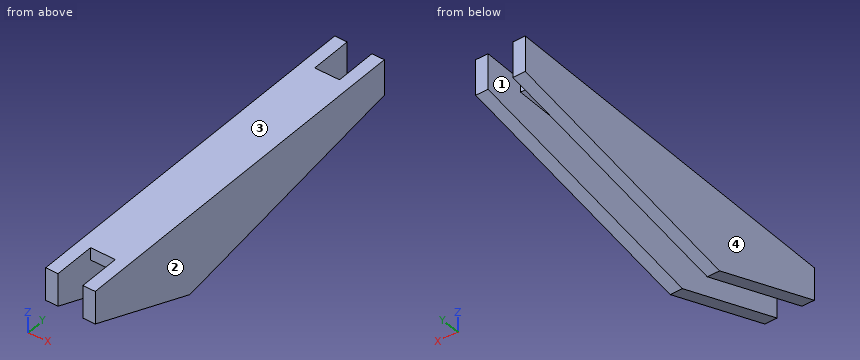
Autodesk Inventor part; units mm, degrees
ref_plane "YZ Plane" through (0, 0, 0) normal (1, 0, 0) x (0, 1, 0)
ref_plane "XZ Plane" through (0, 0, 0) normal (0, 1, 0) x (-1, 0, 0)
ref_plane "XY Plane" through (0, 0, 0) normal (0, 0, 1) x (1, 0, 0)
sketch "BoundingBox" plane through (0, 0, 0) normal (1, 0, 0) x (0, 1, 0)
  line L0 (434.8115, 24.0504) -> (-18, 24.0504)
  line L1 (-18, 24.0504) -> (-18, -15.6719)
  line L2 (-18, -15.6719) -> (130.2861, -72.3729)
  line L3 (130.2861, -72.3729) -> (434.8115, -19.2646)
  line L4 (434.8115, -19.2646) -> (434.8115, 24.0504)
  point P0 (0, 0)
  point P1 (417.3115, 0.6447)
  point P2 (-18, 4.1892)
  dimension "d5" = 24.0504
  dimension "d6" = 4.1893
  dimension "d7" = 110.926
  dimension "d8" = 452.8115
  dimension "d9" = 39.7223
  dimension "d10" = 43.315
  dimension "d11" = 99.893
  dimension "d12" = 56.7009
  dimension "d13" = 17.5
  dimension "d14" = 23.4057
extrude "BoundingBoxFeature" add sketch "BoundingBox" along normal mid plane 60
sketch "ForearmSpace" plane through (0, 0, 0) normal (0, 0, 1) x (1, 0, 0)
  line L0 (15, 142.9861) -> (-15, 142.9861)
  line L1 (-15, 142.9861) -> (-15, 434.8115)
  line L2 (-15, 434.8115) -> (15, 434.8115)
  line L3 (15, 434.8115) -> (15, 142.9861)
  line L4 (-30, 434.8115) -> (30, 434.8115)
  line L5 (0, -86.9623) -> (0, 521.7738)
  line L6 (30, 130.2861) -> (30, 434.8115)
  line L7 (-30, 130.2861) -> (30, 130.2861)
  line L8 (-30, 434.8115) -> (-30, 130.2861)
  line L9 (15, 142.9861) -> (-15, 142.9861)
  line L10 (-15, 142.9861) -> (-15, -18)
  line L11 (-15, -18) -> (15, -18)
  line L12 (15, -18) -> (15, 142.9861)
  line L13 (-30, -18) -> (30, -18)
  point P0 (0, 0)
  point P1 (-30, 282.5488)
  point P2 (0, 142.9861)
  dimension "d19" = 12.7
  dimension "d21" = 30
extrude "ForearmCutFeature" cut sketch "ForearmSpace" along normal through all both and the other way through all contours L12 L7 L5 L0 | L0 L5 L2 L3 | L5 L7 L10 L0 | L0 L1 L2 L5 | L12 L11 L5 L7 | L5 L11 L10 L7
sketch "Sketch4" plane through (30, 0, 0) normal (1, 0, 0) x (0, 0, -1)
  line L0 (-24.0504, 434.8115) -> (-24.0504, -18)
  line L1 (-24.0504, 32.8) -> (-9.0504, 32.8)
  line L2 (-9.0504, 32.8) -> (-9.0504, 384.0115)
  line L3 (-9.0504, 384.0115) -> (-24.0504, 384.0115)
  line L4 (-24.0504, 384.0115) -> (-24.0504, 32.8)
  line L5 (-24.0504, -18) -> (15.6719, -18)
  line L6 (19.2646, 434.8115) -> (-24.0504, 434.8115)
  point P0 (0, 0)
  dimension "d25" = 15
  dimension "d26" = 50.8
  dimension "d27" = 50.8
extrude "Extrusion3" add sketch "Sketch4" against normal up to surface (45 mm away)
properties part number "UpperArmBoundingBox"
Build history of the part. All positions in model axes, mm. Face numbers are marked on the shaded views. Give positions to 0.01 mm unless a question says otherwise; leave off trailing zeros. Loops run counter-clockwise (first coordinate to the right, second up) from the corner with the lowest first, then second, coordinate; pieces in that order, holes last. Notation, with made-up numbers: (-7, 55) -> (3, 55) arc R26 cw to (3, 88) -> close; hole circle Ø6 at (-9.75, -2). An arc over 180 degrees is marked (long way). One line per question, with ' | ' between items. Start each with the question number.
1) Probe L1, parallel to X at y = 266.5, z = -20.5; L2, parallel to Z at x = 11.5, y = 371.5; L3, parallel to Z at x = 18, y = 395.5. List the from-to ranges inside material, lowest first.
2) Two-plate mould, pull along X, no slides. Class the marked faces 1, 2, 3 and 4: released by +X, released by -X, zero draft, split by the parting line, or undercut.
3) Pin check, flat tips, straight feed: pin 1 (4 mm diameter, centred on x = -3.5, y = 264, fed in from -Z); pin 2 (12 mm diameter, centred on x = -2.5, z = 15.5, fed in from -Y); pin 3 (8 mm diameter, centred on y = 322, z = -39, fed in from -X); pin 4 (16.5 mm diameter, centred on x = 5, z = 13.5, fed in from +Y). Stop position of each tip, or through.
4) Cut at D-D (y = 177.5). Give the cut face in (x, z), plus the area to 3 significant figures.
5) Cut at A-A (z = -8). Give the cut face in (x, y), plus the area to 3 significant figures.
6) Cut at C-C (x = 20.5). Give the cut face in (y, z).
7) Cut at B-B (z = 16). Give the cut face in (x, y).
Return value:
1) L1: -30 to -15, 15 to 30 | L2: 9.05 to 24.05 | L3: -26.12 to 24.05
2) face 1: undercut | face 2: released by +X | face 3: zero draft | face 4: released by -X
3) pin 1: z = 9.05 | pin 2: y = 32.8 | pin 3: x = -30 | pin 4: y = 384.01
4) outline: (-30, -64.14) -> (-15, -64.14) -> (-15, 9.05) -> (15, 9.05) -> (15, -64.14) -> (30, -64.14) -> (30, 24.05) -> (-30, 24.05) -> close | area: 3,100 mm^2
5) outline: (-30, -18) -> (-15, -18) -> (-15, 434.81) -> (-30, 434.81) -> close; (15, -18) -> (30, -18) -> (30, 434.81) -> (15, 434.81) -> close | area: 13,600 mm^2
6) outline: (-18, -15.67) -> (130.29, -72.37) -> (434.81, -19.26) -> (434.81, 24.05) -> (-18, 24.05) -> close
7) outline: (-30, -18) -> (-15, -18) -> (-15, 32.8) -> (15, 32.8) -> (15, -18) -> (30, -18) -> (30, 434.81) -> (15, 434.81) -> (15, 384.01) -> (-15, 384.01) -> (-15, 434.81) -> (-30, 434.81) -> close
